from build123d import *

# Parameters (mm, degrees)
SKIZZE1_R                       = 2.7
AUFSATZ_LINEAR_AUSTRAGEN1_DEPTH = 2.95
SKIZZE2_R                       = 1.45
AUFSATZ_LINEAR_AUSTRAGEN2_DEPTH = 20
FASE1_SIZE                      = 0.3
SCHNITT_LINEAR_AUSTRAGEN1_DEPTH = 2.5


with BuildPart() as part:
    # Skizze1 → Aufsatz-Linear austragen1 (new body)
    with BuildSketch(Plane.XY):
        Circle(SKIZZE1_R)
    extrude(amount=AUFSATZ_LINEAR_AUSTRAGEN1_DEPTH)

    # Skizze2 → Aufsatz-Linear austragen2 (add)
    with BuildSketch(Plane.XY.offset(2.95)):
        Circle(SKIZZE2_R)
    extrude(amount=AUFSATZ_LINEAR_AUSTRAGEN2_DEPTH)

    # Fase1
    fase1_edges = [part.edges().sort_by_distance(p)[0] for p in [
        (-2.7, 0, 0),
        (-2.7, 0, 2.95),
        (-1.45, 0, 22.95),
    ]]
    chamfer(fase1_edges, length=FASE1_SIZE)

    # Skizze3 → Schnitt-Linear austragen1 (cut)
    with BuildSketch(Plane(origin=(0, 0, 0), x_dir=(-1, 0, 0), z_dir=(0, 0, -1))):
        Polygon((1.25, 0.721687836), (0, 1.443375673), (-1.25, 0.721687836), (-1.25, -0.721687836), (0, -1.443375673), (1.25, -0.721687836), align=None)
    extrude(amount=-SCHNITT_LINEAR_AUSTRAGEN1_DEPTH, mode=Mode.SUBTRACT)


solid = part.part
The listing builds one solid part. Answer for the finished solid, in the listing's coordinates (mm). A direction names the side the tool comes from. Give positions to 0.01 mm unless a question says otherwise; leave off trailing zeros. Write each loop counter-clockwise with the first axis right and the second up, starting at its lowest first coordinate (ties: lowest second). Pieces come first, ordered by that corner, then holes. Notation, with made-up numbers: (19.5, 59.5) - (44.5, 59.5) arc R16 ccw to (44.5, 86.5) - close; hole circle Ø5 at (87.25, 28). An arc over 180 degrees is marked (long way). One line per question, with ' | ' between items. Start each with the question number.
1. For faces 4 (the face through (1.03, -1.03, 0)), 5 (the face through (-1.45, 0.06, 12.66)), 6 (the face through (0, 0, 2.5)), determine the directions among +Z, -Z, +X, -X, +Y, -Y from which every point of the face is accessible in a straight line to the end or side of a thin tool.
2. Straight lines are drawn through the part: line 1 (Z direction, x = -2.35, y = -0.3); line 2 (Y direction, x = 0.05, z = 2); line 3 (Y direction, x = -1.2, z = 1.5). For each, find the intervals that lie inside material, in ascending order.
3. Section A-A, the plane y = 0 is taken. Determine the outline of the cut face in (x, z), then the cut area to 3 significant figures.
4. Determine the mould class of faces 1 (the face through (0, 0, 22.95)), 2 (the face through (-0.585, -2.636, 1.459)), 3 (the face through (0.63, -1.08, 1.23)) for opening direction X: +X half, -X half, draft (parallel to the pull), parting line (faces both ways), or undercut.
5. Section B-B, the plane z = 6 is taken. Determine the outline of the cut face in (x, y).
6. Given P1, Ø2, axis at x = 0.5, z = 10, coming from the +Y side, flat-ended and moving along its own axis, determine where the tip first touches the part or whether it passes through.
Result:
1) face 4: -Z, +X, -X, +Y, -Y | face 5: +Z | face 6: -Z
2) line 1: z = 0 to 2.95 | line 2: y = -2.7 to -1.41, 1.41 to 2.7 | line 3: y = -2.42 to -0.75, 0.75 to 2.42
3) outline: (-2.7, 0.3) - (-2.4, 0) - (-1.25, 0) - (-1.25, 2.5) - (1.25, 2.5) - (1.25, 0) - (2.4, 0) - (2.7, 0.3) - (2.7, 2.65) - (2.4, 2.95) - (1.45, 2.95) - (1.45, 22.65) - (1.15, 22.95) - (-1.15, 22.95) - (-1.45, 22.65) - (-1.45, 2.95) - (-2.4, 2.95) - (-2.7, 2.65) - close | area: 67.4 mm2
4) face 1: draft | face 2: parting line | face 3: undercut
5) outline: circle Ø2.9 at (0, 0)
6) P1: stops at y = 1.45
